Read the model definition and answer for the solid it produces. Units are mm, in the model's axes. A direction names the side the tool comes from. Round coordinates to 2 decimals unless told otherwise and drop trailing zeros. Order: outer loops, then holes, each group sorted by start corner. A loop starts at its lowest first (then second) coordinate and runs counter-clockwise, first axis right, second up. Notation, with made-up numbers: M 14,-14.5 L 72,-14.5 A19 ccw 72,3.5 Z; hole C 33.5,71 d4. An arc over 180 degrees is marked long. Use one line per item in the form item = value. Start each with the question number.
from build123d import *

# Parameters (mm, degrees)
F1_DEPTH = 5.08
F2_R     = 3.048
F3_DEPTH = 5.08
F5_DEPTH = 5.08
F6_W     = 7.62
F6_H     = 15.24
F7_DEPTH = 5.08
F8_R     = 0.762


# Not quite as in the source:
# - a feature names something its author has since deleted; it is built from what else it names


with BuildPart() as f1:
    # F0 (on Top) → F1 (new body)
    with BuildSketch(Plane.XY):
        with BuildLine():
            ThreePointArc((0, -7.62), (-7.62, 0), (0, 7.62))
            Line((0, 7.62), (-17.78, 7.62))
            Line((-17.78, 7.62), (-17.78, -7.62))
            Line((-17.78, -7.62), (0, -7.62))
        make_face()
        with BuildLine():
            Line((0, -7.62), (0, 7.62))
            ThreePointArc((0, 7.62), (-7.62, 0), (0, -7.62))
        make_face()
        with BuildLine():
            ThreePointArc((0, -7.62), (5.3881536726, -5.3881536726), (7.62, 0))
            ThreePointArc((7.62, 0), (5.3881536726, 5.3881536726), (0, 7.62))
            Line((0, 7.62), (0, -7.62))
        make_face()
    extrude(amount=F1_DEPTH)

    # F2 (on face) → F3 (join)
    with BuildSketch(Plane.XY.offset(5.08)):
        Circle(F2_R)
    extrude(amount=F3_DEPTH)

    # F4 (on face) → F5 (join)
    with BuildSketch(Plane.XY.offset(10.16)):
        with BuildLine():
            ThreePointArc((0, -7.62), (5.3881536726, -5.3881536726), (7.62, 0))
            ThreePointArc((7.62, 0), (5.3881536726, 5.3881536726), (0, 7.62))
            Line((0, 7.62), (0, 3.048))
            ThreePointArc((0, 3.048), (2.1552614691, 2.1552614691), (3.048, 0))
            ThreePointArc((3.048, 0), (2.1552614691, -2.1552614691), (0, -3.048))
            Line((0, -3.048), (0, -7.62))
        make_face()
        with BuildLine():
            Line((0, 3.048), (0, 7.62))
            ThreePointArc((0, 7.62), (-7.62, 0), (0, -7.62))
            Line((0, -7.62), (0, -3.048))
            ThreePointArc((0, -3.048), (-3.048, 0), (0, 3.048))
        make_face()
        with BuildLine():
            ThreePointArc((0, -7.62), (-7.62, 0), (0, 7.62))
            Line((0, 7.62), (-17.78, 7.62))
            Line((-17.78, 7.62), (-17.78, -7.62))
            Line((-17.78, -7.62), (0, -7.62))
        make_face()
        with BuildLine():
            ThreePointArc((0, -7.62), (5.3881536726, -5.3881536726), (7.62, 0))
            ThreePointArc((7.62, 0), (5.3881536726, 5.3881536726), (0, 7.62))
            Line((0, 7.62), (0, -7.62))
        make_face()
        with BuildLine():
            Line((0, -7.62), (0, 7.62))
            ThreePointArc((0, 7.62), (-7.62, 0), (0, -7.62))
        make_face()
    extrude(amount=F5_DEPTH)

    # F6 (on face) → F7 (join)
    with BuildSketch(Plane.XY.offset(5.08)):
        with Locations((-13.97, 0)):
            Rectangle(F6_W, F6_H)
    extrude(amount=F7_DEPTH)

    # F8
    f8_edges = [f1.edges().sort_by_distance(p)[0] for p in [
        (-8.89, 7.62, 0),
        (7.62, 0, 0),
        (-8.89, -7.62, 0),
        (7.62, 0, 15.24),
        (-17.78, 7.62, 7.62),
        (-17.78, 0, 0),
        (-17.78, -7.62, 7.62),
        (-17.78, 0, 15.24),
        (7.62, 0, 5.08),
        (7.62, 0, 10.16),
        (-10.16, -7.62, 7.62),
        (-10.16, 7.62, 7.62),
        (-8.89, 7.62, 15.24),
        (-8.89, -7.62, 15.24),
        (-5.08, -7.62, 5.08),
        (-5.08, 7.62, 5.08),
        (-5.08, -7.62, 10.16),
        (-5.08, 7.62, 10.16),
    ]]
    fillet(f8_edges, radius=F8_R)


solid = f1.part
Item 1: For a pull along Z with two mould halves and no side action, classify faces 3 (the flat face through (-10.16, 0, 8)), 4 (the flat face through (-5, 0, 15.24)), 5 (the flat face through (-5, 0, 0)) as pulls with the +Z half, pulls with the -Z half, needs draft (parallel to the pull), parting line crosses it, or undercut.
Item 2: A tool of negligible diameter and unlimited length cuts with its end or side. For faces 1 (the flat face through (-4, 0, 10.16)), 2 (the flat face through (-12, -7.62, 8)), from which of +Z, -Z, +X, -X, +Y, -Y can it reach the whole face along a straight path? Write none if from no direction.
Item 3: Section C-C (x = -1.75) is taken. Write down the section's boundary in (y, z), and give its area (3 significant figures).
Item 4: Find the intervals of material crossed by L1, parallel to Z at x = -10, y = 5.75; L2, parallel to X at y = -5, z = 9; L3, parallel to X at y = -1, z = 5.5, in increasing order. Write a range as [from, to].
Item 5: Section A-A (z = 6) is taken. Write down the section's boundary in (x, y).
Item 6: Section B-B (z = 3.5) is taken. Write down the section's boundary in (x, y).
Item 7: Given P1, Ø3, axis at x = 2.5, z = 6, coming from the +Y side; P2, Ø5.5, axis at y = 3, z = 7.5, coming from the +X side, each flat-ended and moving along its own axis, determine where each tip first touches the part or whether it passes through.
The answers:
q1.face_3 = undercut
q1.face_4 = pulls with the +Z half
q1.face_5 = pulls with the -Z half
q2.face_1 = none
q2.face_2 = +Z, -Z, +X, -X, -Y
q3.outline = M -7.62,0.76 A0.76 ccw -6.86,0 L 6.86,0 A0.76 ccw 7.62,0.76 L 7.62,4.32 A0.76 ccw 6.86,5.08 L 2.5,5.08 L 2.5,10.16 L 6.86,10.16 A0.76 ccw 7.62,10.92 L 7.62,14.48 A0.76 ccw 6.86,15.24 L -6.86,15.24 A0.76 ccw -7.62,14.48 L -7.62,10.92 A0.76 ccw -6.86,10.16 L -2.5,10.16 L -2.5,5.08 L -6.86,5.08 A0.76 ccw -7.62,4.32 Z
q3.area = 179 mm²
q4.L1 = [0, 5.08], [10.16, 15.24]
q4.L2 = [-17.78, -10.16]
q4.L3 = [-17.78, -10.16], [-2.88, 2.88]
q5.outline = M -17.78,-6.86 A0.76 ccw -17.02,-7.62 L -10.92,-7.62 A0.76 ccw -10.16,-6.86 L -10.16,6.86 A0.76 ccw -10.92,7.62 L -17.02,7.62 A0.76 ccw -17.78,6.86 Z; C 0,0 d6.1
q6.outline = M -17.78,-6.86 A0.76 ccw -17.02,-7.62 L 0,-7.62 A7.62 ccw 0,7.62 L -17.02,7.62 A0.76 ccw -17.78,6.86 Z
q7.P1 = 7.31
q7.P2 = 7.05
